Can you work these out from the model? Positions are in its coordinate system, mm. A direction names the side the tool comes from. Coordinates: 2 decimals unless noted, no trailing zeros. Order: outer loops, then holes, each group sorted by start corner. A loop starts at its lowest first (then second) coordinate and runs counter-clockwise, first axis right, second up. Notation, with made-up numbers: (26, -6) - (39, -6) arc R31 ccw to (39, 22) - close; hole circle Ø4 at (59, 40.5). An arc over 180 degrees is marked (long way). Return JSON: item names as keys, results as strings. Group by question number.
1) Which directions (+Z, -Z, +X, -X, +Y, -Y) give clear straight access to the entire face, cutting with the end or side of a thin tool? Please do faces 1 (the face through (-0.69, 3.1, 14.86)), 2 (the face through (4.315, 2.538, 30.641)).
2) Imagine slicing it at B-B (y = 0.5). Write out the boundary of the cut face in (x, z).
3) For pin 1 Ø2 at (x, z) = (-3.5, 17.5) entering from +Y; pin 2 Ø6 at (y, z) = (-2.5, 10) entering from +X (3 decimals); pin 3 Ø6 at (y, z) = (-3.5, 19) entering from -X, each with a flat end and sliding along its axis, tell me the tip position at first contact or that it passes through.
4) Imagine slicing it at D-D (y = -3.75). Write out the boundary of the cut face in (x, z), and give its area (3 significant figures).
5) If I drill on line 1 along Z through (x, y) = (-4, -1.5); line 2 along X through (y, z) = (-0.25, 21); line 3 along X through (y, z) = (-1, 21), over which ranges is the centre line in solid material (lowest first)?
6) Imagine slicing it at C-C (z = 15.5). Write out the boundary of the cut face in (x, y) (3 decimals).
7) Imagine slicing it at A-A (x = 0). Write out the boundary of the cut face in (y, z) (3 decimals).
Autodesk Inventor part; units mm, degrees
ref_plane "YZ Plane" through (0, 0, 0) normal (1, 0, 0) x (0, 1, 0)
ref_plane "XZ Plane" through (0, 0, 0) normal (0, 1, 0) x (-1, 0, 0)
ref_plane "XY Plane" through (0, 0, 0) normal (0, 0, 1) x (1, 0, 0)
sketch "Sketch1" plane through (0, 0, 0) normal (0, 0, 1) x (1, 0, 0)
  circle A0 centre (0, 0) radius 3.175
  dimension "d0" = 6.35
extrude "Extrusion1" add sketch "Sketch1" along normal blind 30.148
sketch "Sketch2" plane through (0, 0, 30.148) normal (0, 0, 1) x (1, 0, 0)
  line L0 (5.7808, 0) -> (2.8904, -5.0064)
  line L1 (2.8904, -5.0064) -> (-2.8904, -5.0064)
  line L2 (-2.8904, -5.0064) -> (-5.7808, 0)
  line L3 (-5.7808, 0) -> (-2.8904, 5.0064)
  line L4 (-2.8904, 5.0064) -> (2.8904, 5.0064)
  line L5 (2.8904, 5.0064) -> (5.7808, 0)
  point P0 (0, 0)
  point P1 (0, 0)
extrude "Extrusion2" add sketch "Sketch2" along normal blind 1
thread "Thread1"
properties part number "Pedal Bolt Outside Right"
Calculated:
{
 "1": {"face 1": "-Z", "face 2": "+Z, -Z, +X, +Y"},
 "2": {"outline": "(-5.49, 30.15) - (-3.14, 30.15) - (-3.14, 0) - (3.14, 0) - (3.14, 30.15) - (5.49, 30.15) - (5.49, 31.15) - (-5.49, 31.15) - close"},
 "3": {"pin 1": "y = 1.96", "pin 2": "x = 3.175", "pin 3": "x = -3.14"},
 "4": {"outline": "(-3.62, 30.15) - (3.62, 30.15) - (3.62, 31.15) - (-3.62, 31.15) - close", "area": "7.23 mm2"},
 "5": {"line 1": "30.15 to 31.15", "line 2": "-3.17 to 3.17", "line 3": "-3.01 to 3.01"},
 "6": {"outline": "circle Ø6.35 at (0, 0)"},
 "7": {"outline": "(-5.006, 30.148) - (-3.175, 30.148) - (-3.175, 0) - (3.175, 0) - (3.175, 30.148) - (5.006, 30.148) - (5.006, 31.148) - (-5.006, 31.148) - close"}
}
